from build123d import *

# Parameters (mm, degrees)
SKETCH1_W      = 9.525
SKETCH1_H      = 60.325
SKETCH1_R      = 1.5875
EXTRUDE1_DEPTH = 1.4986
FILLET1_R      = 3.175


with BuildPart() as part:
    # Sketch1 → Extrude1 (new body, symmetric)
    with BuildSketch(Plane(origin=(0, 0, 0), x_dir=(0, 0, -1), z_dir=(1, 0, 0))):
        with Locations((0, 25.4)):
            Rectangle(SKETCH1_W, SKETCH1_H)
        Circle(SKETCH1_R, mode=Mode.SUBTRACT)
        with Locations((0, 50.8)):
            Circle(SKETCH1_R, mode=Mode.SUBTRACT)
    extrude(amount=EXTRUDE1_DEPTH, both=True)

    # Fillet1
    fillet1_edges = [part.edges().sort_by_distance(p)[0] for p in [
        (0, 55.5625, 4.7625),
        (0, 55.5625, -4.7625),
    ]]
    fillet(fillet1_edges, radius=FILLET1_R)


solid = part.part
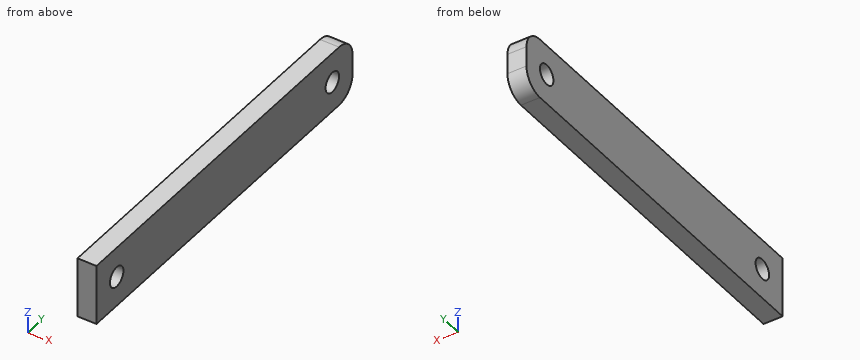
Geometry: final body of the model. Coordinates: model frame, mm. Give positions to 0.01 mm unless a question says otherwise; leave off trailing zeros. Write each loop counter-clockwise with the first axis right and the second up, starting at its lowest first coordinate (ties: lowest second). Pieces come first, ordered by that corner, then holes. Notation, with made-up numbers: M 68,-36.75 L 104,-36.75 A18 cw 104,-14.75 Z; hole C 62,-15.5 d8. An arc over 180 degrees is marked long. Answer in a Markdown table with one row per item. Add a question column.
(1) Section D-D on z = 4. Return loops of the section in (x, y).
(2) Section A-A on z = 0. Return loops of the section in (x, y).
(3) Section B-B on x = -0.55. State how many separate pieces and enclosed holes the cut face has, and give its area (3 significant figures).
(4) Section C-C on y = 0. Return loops of the section in (x, z).
(5) Ray query, line 1 (Y direction, x = 0.4, z = 0); line 2 (Y direction, x = 1.25, z = -1); line 3 (Z direction, x = 0, y = -0.5). Return the intervals inside material, ascending.
Result set:
| question | item | result |
|---|---|---|
| 1 | outline | M -1.5,-4.76 L 1.5,-4.76 L 1.5,54.45 L -1.5,54.45 Z |
| 2 | outline | M -1.5,-4.76 L 1.5,-4.76 L 1.5,-1.59 L -1.5,-1.59 Z; M -1.5,1.59 L 1.5,1.59 L 1.5,49.21 L -1.5,49.21 Z; M -1.5,52.39 L 1.5,52.39 L 1.5,55.56 L -1.5,55.56 Z |
| 3 | separate pieces | 1 |
| 3 | enclosed holes | 2 |
| 3 | area | 554 mm^2 |
| 4 | outline | M -1.5,-4.76 L 1.5,-4.76 L 1.5,-1.59 L -1.5,-1.59 Z; M -1.5,1.59 L 1.5,1.59 L 1.5,4.76 L -1.5,4.76 Z |
| 5 | line 1 | y = -4.76 to -1.59, 1.59 to 49.21, 52.39 to 55.56 |
| 5 | line 2 | y = -4.76 to -1.23, 1.23 to 49.57, 52.03 to 55.56 |
| 5 | line 3 | z = -4.76 to -1.51, 1.51 to 4.76 |
